from build123d import *

# Parameters (mm, degrees)
SKETCH1_W             = 76.2
SKETCH1_H             = 76.2
BOSS_EXTRUDE1_DEPTH   = 1.5875
F_8_CLEARANCE_HOLE1_D = 4.3053
SKETCH4_W             = 101.6
SKETCH4_H             = 101.6
CUT_EXTRUDE1_DEPTH    = 54.975


with BuildPart() as part:
    # Sketch1 → Boss-Extrude1 (new, symmetric)
    with BuildSketch(Plane(origin=(0, 0, 0), x_dir=(0, 0, -1), z_dir=(1, 0, 0))):
        Rectangle(SKETCH1_W, SKETCH1_H)
    extrude(amount=BOSS_EXTRUDE1_DEPTH, both=True)

    # #8 Clearance Hole1 (through all)
    with Locations(Plane(origin=(1.5875, 0, 0), x_dir=(0, 0, -1), z_dir=(1, 0, 0))):
        with Locations((-25.4, 25.4), (-25.4, 0), (25.4, 25.4), (0, 0), (25.4, 0), (0, -25.4), (25.4, -25.4)):
            Hole(F_8_CLEARANCE_HOLE1_D / 2)

    # Sketch4 → Cut-Extrude1 (cut, through all)
    with BuildSketch(Plane(origin=(1.5875, 0, 0), x_dir=(0, 0, -1), z_dir=(1, 0, 0))):
        Rectangle(SKETCH4_W, SKETCH4_H)
        with BuildLine():
            Line((-38.1, 0), (-38.1, 25.4))
            ThreePointArc((-38.1, 25.4), (-34.380256121, 34.380256121), (-25.4, 38.1))
            Line((-25.4, 38.1), (25.4, 38.1))
            ThreePointArc((25.4, 38.1), (34.380256121, 34.380256121), (38.1, 25.4))
            Line((38.1, 25.4), (38.1, -25.4))
            ThreePointArc((38.1, -25.4), (34.380256121, -34.380256121), (25.4, -38.1))
            Line((25.4, -38.1), (0, -38.1))
            ThreePointArc((0, -38.1), (-8.980256121, -34.380256121), (-12.7, -25.4))
            ThreePointArc((-12.7, -25.4), (-16.419743879, -16.419743879), (-25.4, -12.7))
            ThreePointArc((-25.4, -12.7), (-34.380256121, -8.980256121), (-38.1, 0))
        make_face(mode=Mode.SUBTRACT)
    extrude(amount=-CUT_EXTRUDE1_DEPTH, mode=Mode.SUBTRACT)


solid = part.part
CAD build for the part. Positions are in the model's coordinates, mm. Round coordinates to 2 decimals unless told otherwise and drop trailing zeros. Loops run counter-clockwise (first coordinate to the right, second up) from the corner with the lowest first, then second, coordinate; pieces in that order, holes last. Notation, with made-up numbers: (76, -11.5) - (135, -11.5) arc R21 cw to (135, 25.5) - close; hole circle Ø10 at (-28.5, 87.5). An arc over 180 degrees is marked (long way). Put each result on its own line as item: value.
1. Slice it at C-C on z = 19.5. List the corners of the cut face in (x, y), and give its area (3 significant figures).
Geometry check:
outline: (-1.59, -14.15) - (1.59, -14.15) - (1.59, 38.1) - (-1.59, 38.1) - close
area: 166 mm²
2. Slice it at A-A on x = 0.1. List the corners of the cut face in (y, z), and give its area (3 significant figures).
Geometry check:
outline: (-38.1, -25.4) arc R12.7 ccw to (-25.4, -38.1) - (25.4, -38.1) arc R12.7 ccw to (38.1, -25.4) - (38.1, 25.4) arc R12.7 ccw to (25.4, 38.1) - (0, 38.1) arc R12.7 ccw to (-12.7, 25.4) arc R12.7 cw to (-25.4, 12.7) arc R12.7 ccw to (-38.1, 0) - close; hole circle Ø4.31 at (-25.4, -25.4); hole circle Ø4.31 at (-25.4, 0); hole circle Ø4.31 at (0, -25.4); hole circle Ø4.31 at (0, 0); hole circle Ø4.31 at (0, 25.4); hole circle Ø4.31 at (25.4, -25.4); hole circle Ø4.31 at (25.4, 25.4)
area: 4,920 mm²
3. Slice it at D-D on y = -31. List the corners of the cut face in (x, z).
Geometry check:
outline: (-1.59, -36.8) - (1.59, -36.8) - (1.59, 11.4) - (-1.59, 11.4) - close
4. Pin check, flat tip, straight feed: P1, Ø2.5, axis at y = 25.4, z = 25.4, coming from the -X side. Stop position of the tip, or through.
Geometry check:
P1: through
5. Slice it at B-B on y = 24.5. List the corners of the cut face in (x, z), and give its area (3 significant figures).
Geometry check:
outline: (-1.59, -38.1) - (1.59, -38.1) - (1.59, -27.36) - (-1.59, -27.36) - close; (-1.59, -23.44) - (1.59, -23.44) - (1.59, 23.44) - (-1.59, 23.44) - close; (-1.59, 27.36) - (1.59, 27.36) - (1.59, 38.1) - (-1.59, 38.1) - close
area: 217 mm²
6. Two-plate mould, pull along Y, no slides. Class faces 1 (the cylindrical face through (-0.02, 23.49, -24.41)), 2 (the flat face through (0, 13, 38.1)), 3 (the flat face through (0, 38.1, 0)): released by +Y, released by -Y, zero draft, split by the parting line, or undercut.
Geometry check:
face 1: undercut
face 2: zero draft
face 3: released by +Y
7. Wall check: line 1 (Y direction, x = -0.65, z = -25.4); line 2 (Y direction, x = 0.3, z = 0); line 3 (Y direction, x = 0.9, z = 25.4). Give the ranges that are in metal, low to high.
Geometry check:
line 1: -38.1 to -27.55, -23.25 to -2.15, 2.15 to 23.25, 27.55 to 38.1
line 2: -38.1 to -27.55, -23.25 to -2.15, 2.15 to 38.1
line 3: -12.7 to -2.15, 2.15 to 23.25, 27.55 to 38.1
